Check sheet for the modelled part. Datum: model origin and axes. Units: mm. Coordinates: 2 decimals unless noted, no trailing zeros. Write each loop counter-clockwise with the first axis right and the second up, starting at its lowest first coordinate (ties: lowest second). Pieces come first, ordered by that corner, then holes. Notation, with made-up numbers: M 40,39 L 90,39 A7 ccw 90,46 Z; hole C 71,35.5 d1. An arc over 180 degrees is marked long. Answer as CSV lines item,"result". Start each with the question number.
Q1. Thickness scan on line 1 along X through (y, z) = (66.5, 7.5); line 2 along Y through (x, z) = (-99, 2.75); line 3 along X through (y, z) = (61, 9). Record the ranges inside material, lowest first. Write a range as from..to.
Q2. Sectioned sample at B-B, the plane z = 9.25. Count the separate pieces of the cut face and the enclosed holes in it, then the cut area to 3 significant figures.
Q3. Depth check by flat-ended pin: pin 1 Ø4 at (y, z) = (-38.5, 10.5) entering from -X; pin 2 Ø13 at (x, y) = (74.5, -43.5) entering from +Z; pin 3 Ø6 at (y, z) = (-51, 9.5) entering from +X. Enter the tip coordinate at first touch or a pass-through.
Q4. Sectioned sample at A-A, the plane x = -102.5. Record the cut outline in (y, z).
from build123d import *

# Parameters (mm, degrees)
F1_DEPTH = 12.7
F2_R     = 12.6899466908
F3_DEPTH = 6.35
F4_R     = 13.0916621451
F5_DEPTH = 6.35
F6_R     = 13.1338166207
F7_DEPTH = 6.35
F8_R     = 12.797635225
F9_DEPTH = 6.35


with BuildPart() as f1:
    # F0 (on Top) → F1 (new body)
    with BuildSketch(Plane.XY):
        with BuildLine():
            add(Edge.make_bspline(
                [(-97.9790315032, 57.3151484132), (-94.8917277119, 49.2634504814), (-91.8044239206, 41.2117525495), (-89.3433409519, 33.1833022823)],
                knots=[0, 0, 0, 0, 0.2258221369, 0.2258221369, 0.2258221369, 0.2258221369], degree=3))
            ThreePointArc((-89.3433409519, 33.1833022823), (-79.1894484696, 39.8832030713), (-73.2684448417, 50.5101461484))
            add(Edge.make_bspline(
                [(-97.9790315032, 57.3151484132), (-89.7678150487, 54.9705923246), (-81.5565985942, 52.6260362361), (-73.2684448417, 50.5101461484)],
                knots=[0, 0, 0, 0, 0.1532150424, 0.1532150424, 0.1532150424, 0.1532150424], degree=3))
        make_face()
        with BuildLine():
            Line((-72.348558449, 57.3151484132), (-97.9790315032, 57.3151484132))
            add(Edge.make_bspline(
                [(-97.9790315032, 57.3151484132), (-89.7678150487, 54.9705923246), (-81.5565985942, 52.6260362361), (-73.2684448417, 50.5101461484)],
                knots=[0, 0, 0, 0, 0.1532150424, 0.1532150424, 0.1532150424, 0.1532150424], degree=3))
            ThreePointArc((-73.2684448417, 50.5101461484), (-72.5795711294, 53.8817009183), (-72.348558449, 57.3151484132))
        make_face()
        with BuildLine():
            Line((-97.9790315032, 57.3151484132), (-97.9790315032, 31.684675359))
            ThreePointArc((-97.9790315032, 31.684675359), (-93.5966510441, 32.0621111604), (-89.3433409519, 33.1833022823))
            add(Edge.make_bspline(
                [(-97.9790315032, 57.3151484132), (-94.8917277119, 49.2634504814), (-91.8044239206, 41.2117525495), (-89.3433409519, 33.1833022823)],
                knots=[0, 0, 0, 0, 0.2258221369, 0.2258221369, 0.2258221369, 0.2258221369], degree=3))
        make_face()
        with BuildLine():
            ThreePointArc((-72.348558449, 57.3151484132), (-116.1025128048, 75.4386297148), (-97.9790315032, 31.684675359))
            Line((-97.9790315032, 31.684675359), (-97.9790315032, 57.3151484132))
            Line((-97.9790315032, 57.3151484132), (-72.348558449, 57.3151484132))
        make_face()
        with BuildLine():
            Line((-97.9790315032, -22.6032967451), (-97.9790315032, -48.1273792684))
            add(Edge.make_bspline(
                [(-89.1568913198, -24.1764162139), (-91.6474722391, -32.1767811704), (-94.8132518711, -40.1520802194), (-97.9790315032, -48.1273792684)],
                knots=[0.7697468516, 0.7697468516, 0.7697468516, 0.7697468516, 1, 1, 1, 1], degree=3))
            ThreePointArc((-89.1568913198, -24.1764162139), (-93.4983824911, -22.9996540812), (-97.9790315032, -22.6032967451))
        make_face()
        with BuildLine():
            add(Edge.make_bspline(
                [(-97.9790315032, -48.1273792684), (-89.8692523818, -45.5267859125), (-81.7594732605, -42.9261925567), (-73.6038589741, -40.5557379118)],
                knots=[0, 0, 0, 0, 0.1468762855, 0.1468762855, 0.1468762855, 0.1468762855], degree=3))
            Line((-97.9790315032, -48.1273792684), (-72.4549489799, -48.1273792684))
            ThreePointArc((-72.4549489799, -48.1273792684), (-72.7438110385, -44.2982231274), (-73.6038589741, -40.5557379118))
        make_face()
        with BuildLine():
            add(Edge.make_bspline(
                [(-89.1568913198, -24.1764162139), (-91.6474722391, -32.1767811704), (-94.8132518711, -40.1520802194), (-97.9790315032, -48.1273792684)],
                knots=[0.7697468516, 0.7697468516, 0.7697468516, 0.7697468516, 1, 1, 1, 1], degree=3))
            add(Edge.make_bspline(
                [(-97.9790315032, -48.1273792684), (-89.8692523818, -45.5267859125), (-81.7594732605, -42.9261925567), (-73.6038589741, -40.5557379118)],
                knots=[0, 0, 0, 0, 0.1468762855, 0.1468762855, 0.1468762855, 0.1468762855], degree=3))
            ThreePointArc((-73.6038589741, -40.5557379118), (-79.4699543341, -30.5520314482), (-89.1568913198, -24.1764162139))
        make_face()
        with BuildLine():
            Line((-72.4549489799, -48.1273792684), (-97.9790315032, -48.1273792684))
            Line((-97.9790315032, -48.1273792684), (-97.9790315032, -22.6032967451))
            ThreePointArc((-97.9790315032, -22.6032967451), (-116.027283339, -66.1756311042), (-72.4549489799, -48.1273792684))
        make_face()
        with BuildLine():
            ThreePointArc((69.2940983232, -24.2495217193), (59.3934172366, -30.9551926113), (53.638077891, -41.436870774))
            add(Edge.make_bspline(
                [(53.638077891, -41.436870774), (61.8198164822, -43.5633793037), (70.0325232507, -45.845379286), (78.2452300191, -48.1273792684)],
                knots=[0.8679259668, 0.8679259668, 0.8679259668, 0.8679259668, 1, 1, 1, 1], degree=3))
            add(Edge.make_bspline(
                [(78.2452300191, -48.1273792684), (75.0007191566, -40.2161005478), (71.7562082941, -32.3048218271), (69.2940983232, -24.2495217193)],
                knots=[0, 0, 0, 0, 0.2420801973, 0.2420801973, 0.2420801973, 0.2420801973], degree=3))
        make_face()
        with BuildLine():
            add(Edge.make_bspline(
                [(78.2452300191, -48.1273792684), (75.0007191566, -40.2161005478), (71.7562082941, -32.3048218271), (69.2940983232, -24.2495217193)],
                knots=[0, 0, 0, 0, 0.2420801973, 0.2420801973, 0.2420801973, 0.2420801973], degree=3))
            Line((78.2452300191, -48.1273792684), (78.2452300191, -22.6268922187))
            ThreePointArc((78.2452300191, -22.6268922187), (73.6967224305, -23.0358285294), (69.2940983232, -24.2495217193))
        make_face()
        with BuildLine():
            ThreePointArc((53.638077891, -41.436870774), (52.9690633404, -44.752436632), (52.7447429694, -48.1273792684))
            Line((52.7447429694, -48.1273792684), (78.2452300191, -48.1273792684))
            add(Edge.make_bspline(
                [(53.638077891, -41.436870774), (61.8198164822, -43.5633793037), (70.0325232507, -45.845379286), (78.2452300191, -48.1273792684)],
                knots=[0.8679259668, 0.8679259668, 0.8679259668, 0.8679259668, 1, 1, 1, 1], degree=3))
        make_face()
        with BuildLine():
            Line((78.2452300191, -48.1273792684), (52.7447429694, -48.1273792684))
            ThreePointArc((52.7447429694, -48.1273792684), (78.2452300191, -73.6278663181), (103.7457170688, -48.1273792684))
            ThreePointArc((103.7457170688, -48.1273792684), (96.2767973355, -30.095811952), (78.2452300191, -22.6268922187))
            Line((78.2452300191, -22.6268922187), (78.2452300191, -48.1273792684))
        make_face()
        with BuildLine():
            add(Edge.make_bspline(
                [(70.2099663174, 32.740651796), (72.5324991188, 40.8666400762), (75.388864569, 49.0908942447), (78.2452300191, 57.3151484132)],
                knots=[0.7809669753, 0.7809669753, 0.7809669753, 0.7809669753, 1, 1, 1, 1], degree=3))
            ThreePointArc((70.2099663174, 32.740651796), (74.1769173352, 31.782420814), (78.2452300191, 31.4603355779))
            Line((78.2452300191, 31.4603355779), (78.2452300191, 57.3151484132))
        make_face()
        with BuildLine():
            add(Edge.make_bspline(
                [(53.0309728344, 51.5956570573), (61.4062012949, 53.4144058383), (69.825715657, 55.3647771258), (78.2452300191, 57.3151484132)],
                knots=[0.8678396009, 0.8678396009, 0.8678396009, 0.8678396009, 1, 1, 1, 1], degree=3))
            ThreePointArc((53.0309728344, 51.5956570573), (59.1334413627, 39.9021968799), (70.2099663174, 32.740651796))
            add(Edge.make_bspline(
                [(70.2099663174, 32.740651796), (72.5324991188, 40.8666400762), (75.388864569, 49.0908942447), (78.2452300191, 57.3151484132)],
                knots=[0.7809669753, 0.7809669753, 0.7809669753, 0.7809669753, 1, 1, 1, 1], degree=3))
        make_face()
        with BuildLine():
            Line((78.2452300191, 57.3151484132), (52.3904171839, 57.3151484132))
            ThreePointArc((52.3904171839, 57.3151484132), (52.5510551244, 54.4375238324), (53.0309728344, 51.5956570573))
            add(Edge.make_bspline(
                [(53.0309728344, 51.5956570573), (61.4062012949, 53.4144058383), (69.825715657, 55.3647771258), (78.2452300191, 57.3151484132)],
                knots=[0.8678396009, 0.8678396009, 0.8678396009, 0.8678396009, 1, 1, 1, 1], degree=3))
        make_face()
        with BuildLine():
            ThreePointArc((104.1000428543, 57.3151484132), (78.2452300191, 83.1699612484), (52.3904171839, 57.3151484132))
            Line((52.3904171839, 57.3151484132), (78.2452300191, 57.3151484132))
            Line((78.2452300191, 57.3151484132), (78.2452300191, 31.4603355779))
            ThreePointArc((78.2452300191, 31.4603355779), (96.5273435012, 39.0330349311), (104.1000428543, 57.3151484132))
        make_face()
        with BuildLine():
            add(Edge.make_bspline(
                [(-89.3433409519, 33.1833022823), (-86.3089203393, 23.2845319899), (-82.2407796779, 4.0159084283), (-86.2851127622, -14.9515496945), (-89.1568913198, -24.1764162139)],
                knots=[0.2258221369, 0.2258221369, 0.2258221369, 0.2258221369, 0.5042521434, 0.7697468516, 0.7697468516, 0.7697468516, 0.7697468516], degree=3))
            ThreePointArc((-89.1568913198, -24.1764162139), (-79.4699543341, -30.5520314482), (-73.6038589741, -40.5557379118))
            add(Edge.make_bspline(
                [(-73.6038589741, -40.5557379118), (-55.0144907829, -35.1526802602), (-14.4638072494, -26.0907707686), (29.7094018219, -35.2175894809), (53.638077891, -41.436870774)],
                knots=[0.1468762855, 0.1468762855, 0.1468762855, 0.1468762855, 0.4816563834, 0.8679259668, 0.8679259668, 0.8679259668, 0.8679259668], degree=3))
            ThreePointArc((53.638077891, -41.436870774), (59.3934172366, -30.9551926113), (69.2940983232, -24.2495217193))
            add(Edge.make_bspline(
                [(69.2940983232, -24.2495217193), (66.8796393942, -16.350121814), (63.1067862028, 1.895913691), (67.0130764735, 21.5554967842), (70.2099663174, 32.740651796)],
                knots=[0.2420801973, 0.2420801973, 0.2420801973, 0.2420801973, 0.4794752368, 0.7809669753, 0.7809669753, 0.7809669753, 0.7809669753], degree=3))
            ThreePointArc((70.2099663174, 32.740651796), (59.1334413627, 39.9021968799), (53.0309728344, 51.5956570573))
            add(Edge.make_bspline(
                [(-73.2684448417, 50.5101461484), (-55.9796971344, 46.0964864848), (-16.5735995756, 38.4523299071), (27.9976145113, 46.1594602838), (53.0309728344, 51.5956570573)],
                knots=[0.1532150424, 0.1532150424, 0.1532150424, 0.1532150424, 0.4728153168, 0.8678396009, 0.8678396009, 0.8678396009, 0.8678396009], degree=3))
            ThreePointArc((-73.2684448417, 50.5101461484), (-79.1894484696, 39.8832030713), (-89.3433409519, 33.1833022823))
        make_face()
    extrude(amount=F1_DEPTH)

    # F2 (on face) → F3 (cut)
    with BuildSketch(Plane.XY.offset(12.7)):
        with Locations((78.2452300191, 57.3151484132)):
            Circle(F2_R)
    extrude(amount=-F3_DEPTH, mode=Mode.SUBTRACT)

    # F4 (on face) → F5 (cut)
    with BuildSketch(Plane.XY.offset(12.7)):
        with Locations((78.2452300191, -48.1273792684)):
            Circle(F4_R)
    extrude(amount=-F5_DEPTH, mode=Mode.SUBTRACT)

    # F6 (on face) → F7 (cut)
    with BuildSketch(Plane.XY.offset(12.7)):
        with Locations((-97.9790315032, 57.3151484132)):
            Circle(F6_R)
    extrude(amount=-F7_DEPTH, mode=Mode.SUBTRACT)

    # F8 (on face) → F9 (cut)
    with BuildSketch(Plane.XY.offset(12.7)):
        with Locations((-97.9790315032, -48.1273792684)):
            Circle(F8_R)
    extrude(amount=-F9_DEPTH, mode=Mode.SUBTRACT)


solid = f1.part
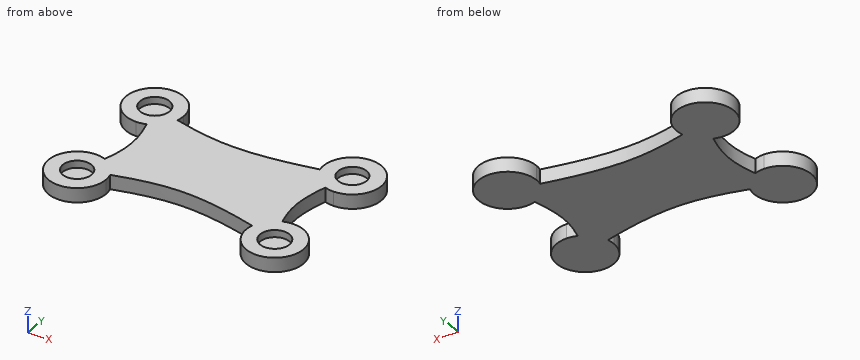
Output:
1,line 1,"x = -121.91..-107.37, -88.59..-74.05, 54.08..69.49, 87..102.41"
1,line 2,"y = -73.63..-22.62, 31.71..82.93"
1,line 3,"x = -123.34..-110.59, -85.37..-72.61, 52.65..66.1, 90.39..103.84"
2,separate pieces,"1"
2,enclosed holes,"4"
2,area,"18,100 mm^2"
3,pin 1,"stops at x = -122.34"
3,pin 2,"stops at z = 6.35"
3,pin 3,"stops at x = 103.75"
4,outline,"M -73.25,0 L -23.01,0 L -23.01,12.7 L -36.15,12.7 L -36.15,6.35 L -60.1,6.35 L -60.1,12.7 L -73.25,12.7 Z; M 32.09,0 L 82.54,0 L 82.54,12.7 L 69.65,12.7 L 69.65,6.35 L 44.98,6.35 L 44.98,12.7 L 32.09,12.7 Z"
